```python
from build123d import *

# Parameters (mm, degrees)
F0_W     = 38.1
F0_H     = 38.1
F1_DEPTH = 1.27
F3_DEPTH = 25.4
F4_R     = 1.5875
F4_W     = 2.54
F4_H     = 8.89
F5_DEPTH = 25.4


with BuildPart() as f1:
    # F0 (on Top) → F1 (new body)
    with BuildSketch(Plane.XY):
        Rectangle(F0_W, F0_H)
    extrude(amount=F1_DEPTH)

    # F2 (on Top) → F3 (cut)
    with BuildSketch(Plane.XY):
        with BuildLine():
            ThreePointArc((-0.518475, 6.200063), (-1.065611, 7.141481), (-2.14087, 7.313076))
            ThreePointArc((-2.14087, 7.313076), (-6.590117, 3.82554), (-7.412157, -1.767578))
            ThreePointArc((-7.412157, -1.767578), (-6.729914, -2.616206), (-5.641081, -2.624462))
            ThreePointArc((-5.641081, -2.624462), (-5.033573, -2.026098), (-4.941438, -1.178385))
            ThreePointArc((-4.941438, -1.178385), (-4.393411, 2.55036), (-1.427246, 4.875384))
            ThreePointArc((-1.427246, 4.875384), (-0.736807, 5.375783), (-0.518475, 6.200063))
        make_face()
        with BuildLine():
            ThreePointArc((5.641081, -2.624462), (6.729914, -2.616206), (7.412157, -1.767578))
            ThreePointArc((7.412157, -1.767578), (6.590117, 3.82554), (2.14087, 7.313076))
            ThreePointArc((2.14087, 7.313076), (1.065611, 7.141481), (0.518475, 6.200063))
            ThreePointArc((0.518475, 6.200063), (0.736807, 5.375783), (1.427246, 4.875384))
            ThreePointArc((1.427246, 4.875384), (4.393411, 2.55036), (4.941438, -1.178385))
            ThreePointArc((4.941438, -1.178385), (5.033573, -2.026098), (5.641081, -2.624462))
        make_face()
        with BuildLine():
            ThreePointArc((-5.126844, -3.524921), (-5.673013, -4.4669), (-5.288787, -5.485721))
            ThreePointArc((-5.288787, -5.485721), (0, -7.62), (5.288787, -5.485721))
            ThreePointArc((5.288787, -5.485721), (5.673013, -4.4669), (5.126844, -3.524921))
            ThreePointArc((5.126844, -3.524921), (4.302789, -3.305743), (3.525858, -3.657147))
            ThreePointArc((3.525858, -3.657147), (0, -5.08), (-3.525858, -3.657147))
            ThreePointArc((-3.525858, -3.657147), (-4.302789, -3.305743), (-5.126844, -3.524921))
        make_face()
    extrude(amount=F3_DEPTH, mode=Mode.SUBTRACT)

    # F4 (on Top) → F5 (cut)
    with BuildSketch(Plane.XY):
        with Locations((13.97, 13.97)):
            Circle(F4_R)
        with Locations((13.97, -13.97)):
            Circle(F4_R)
        with Locations((-13.97, -13.97)):
            Circle(F4_R)
        with Locations((-13.97, 13.97)):
            Circle(F4_R)
        Rectangle(F4_W, F4_H)
    extrude(amount=F5_DEPTH, mode=Mode.SUBTRACT)


solid = f1.part
```
Here's how the part is built. I have some questions about the finished solid (model axes, mm). A direction names the side the tool comes from. Give positions to 0.01 mm unless a question says otherwise; leave off trailing zeros. Loops run counter-clockwise (first coordinate to the right, second up) from the corner with the lowest first, then second, coordinate; pieces in that order, holes last. Notation, with made-up numbers: M 84,19.25 L 139,19.25 A24 ccw 139,52.25 Z; hole C 73.25,34 d2. An arc over 180 degrees is marked long. Return JSON: item names as keys, results as strings.
Item 1: Thinking about a two-plate mould opening in X: for faces 3 (the flat face through (19.05, 0, 1)), 4 (the flat face through (-19.05, 0, 1)), 5 (the cylindrical face through (-4.42, 2.5, 0.63)), which applies, released by +X, released by -X, zero draft, split by the parting line, or undercut?
A:
{"face 3": "released by +X", "face 4": "released by -X", "face 5": "undercut"}
Item 2: Please list where these lines run through material, in increasing order: line 1 (Y direction, x = -13.97, z = 0.6); line 2 (Y direction, x = -13.5, z = 0.7).
A:
{"line 1": "y = -19.05 to -15.56, -12.38 to 12.38, 15.56 to 19.05", "line 2": "y = -19.05 to -15.49, -12.45 to 12.45, 15.49 to 19.05"}
Item 3: Imagine slicing it at B-B on x = 0. List the corners of the cut face in (y, z) for me (3 decimals).
A:
{"outline": "M -19.05,0 L -7.62,0 L -7.62,1.27 L -19.05,1.27 Z; M -5.08,0 L -4.445,0 L -4.445,1.27 L -5.08,1.27 Z; M 4.445,0 L 19.05,0 L 19.05,1.27 L 4.445,1.27 Z"}
Item 4: I'm going to push a flat-ended pin straight in: pin 1 Ø3 at (x, y) = (13.97, 13.97) entering from -Z. Where does the tip first touch, or does it pass through?
A:
{"pin 1": "passes through"}
Item 5: Imagine slicing it at C-C on z = 0.7. State how many separate pieces and enclosed holes the cut face has, then the cut area to 3 significant figures.
A:
{"separate pieces": "1", "enclosed holes": "8", "area": "1,310 mm^2"}
Item 6: Imagine slicing it at D-D on y = 2. List the corners of the cut face in (x, z) for me, then the cut area to 3 significant figures.
A:
{"outline": "M -19.05,0 L -7.35,0 L -7.35,1.27 L -19.05,1.27 Z; M -4.67,0 L -1.27,0 L -1.27,1.27 L -4.67,1.27 Z; M 1.27,0 L 4.67,0 L 4.67,1.27 L 1.27,1.27 Z; M 7.35,0 L 19.05,0 L 19.05,1.27 L 7.35,1.27 Z", "area": "38.3 mm^2"}
Item 7: Imagine slicing it at A-A on y = -13.97. List the corners of the cut face in (x, z) for me.
A:
{"outline": "M -19.05,0 L -15.56,0 L -15.56,1.27 L -19.05,1.27 Z; M -12.38,0 L 12.38,0 L 12.38,1.27 L -12.38,1.27 Z; M 15.56,0 L 19.05,0 L 19.05,1.27 L 15.56,1.27 Z"}
Item 8: On a 3-axis mill with a long thin cutter (end or side, diameter ignored), from which of +Z, -Z, +X, -X, +Y, -Y can I reach the whole of each face in a straight line? I mean faces 1 (the flat face through (-1.27, 0, 1)), 2 (the flat face through (0, -19.05, 1)). Say none if no direction works.
A:
{"face 1": "+Z, -Z", "face 2": "+Z, -Z, +X, -X, -Y"}
